from build123d import *

# Parameters (mm, degrees)
SKETCH_1_W               = 43.2
SKETCH_1_H               = 27.5
EXTRUDE_1_DEPTH          = 2
CUT_EXTRUDE_1_REACH      = 27.683
SKETCH_2_R               = 1.65
CUT_EXTRUDE_2_REACH      = 27.683
MIRROR_2_COPY_1_REACH    = 27.683
MIRROR_2_COPY_1_SKETCH_R = 1.65
MIRROR_2_COPY_2_REACH    = 27.683
CUT_EXTRUDE_3_REACH      = 27.683
SKETCH_4_R               = 4
SKETCH_5_W               = 5
SKETCH_5_H               = 24
EXTRUDE_2_DEPTH          = 19
CUT_EXTRUDE_5_REACH      = 50.159
SKETCH_6_R               = 6
CUT_EXTRUDE_6_REACH      = 35.115
SKETCH_7_R               = 1.65


with BuildPart() as part:
    # 草图1 → 凸台-拉伸1 (new body)
    with BuildSketch(Plane(origin=(0, 0, 0), x_dir=(1, 0, 0), z_dir=(0, 1, 0))):
        Rectangle(SKETCH_1_W, SKETCH_1_H)
    extrude(amount=EXTRUDE_1_DEPTH)

    # 草图2 → 切除-拉伸1 (cut, up to next)
    with BuildSketch(Plane(origin=(0, 2, 0), x_dir=(1, 0, 0), z_dir=(0, 1, 0)), mode=Mode.PRIVATE) as cut_extrude_1_sk1:
        with Locations(Location((-17, 9, 0), (0, 0, 270))):
            Circle(SKETCH_2_R)
    cut_extrude_1_tool1 = extrude(cut_extrude_1_sk1.sketch, amount=-CUT_EXTRUDE_1_REACH, mode=Mode.PRIVATE) & part.part
    cut_extrude_1 = cut_extrude_1_tool1.solids().sort_by_distance((-17, 2, -9))[0]
    add(cut_extrude_1, mode=Mode.SUBTRACT)

    # 草图3 → 切除-拉伸2 (cut, up to next)
    with BuildSketch(Plane(origin=(0, 2, 0), x_dir=(1, 0, 0), z_dir=(0, 1, 0)), mode=Mode.PRIVATE) as cut_extrude_2_sk1:
        with BuildLine():
            Line((-6.788225099, 4.5254834), (-10.033845225, 7.771103525))
            ThreePointArc((-10.033845225, 7.771103525), (-10.033845225, 10.033845225), (-7.771103525, 10.033845225))
            Line((-7.771103525, 10.033845225), (-4.5254834, 6.788225099))
            ThreePointArc((-4.5254834, 6.788225099), (-4.5254834, 4.5254834), (-6.788225099, 4.5254834))
        make_face()
    cut_extrude_2_tool1 = extrude(cut_extrude_2_sk1.sketch, amount=-CUT_EXTRUDE_2_REACH, mode=Mode.PRIVATE) & part.part
    cut_extrude_2 = cut_extrude_2_tool1.solids().sort_by_distance((-7.279664, 2, -7.279664))[0]
    add(cut_extrude_2, mode=Mode.SUBTRACT)

    # 镜向1: 切除-拉伸1, 切除-拉伸2 across plane
    add(cut_extrude_1.mirror(Plane.XY), mode=Mode.SUBTRACT)
    add(cut_extrude_2.mirror(Plane.XY), mode=Mode.SUBTRACT)

    # 镜向2: 切除-拉伸1, 切除-拉伸2 across plane
    add(cut_extrude_1.mirror(Plane(origin=(0, 0, 0), x_dir=(0, 0, 1), z_dir=(1, 0, 0))), mode=Mode.SUBTRACT)
    add(cut_extrude_2.mirror(Plane(origin=(0, 0, 0), x_dir=(0, 0, 1), z_dir=(1, 0, 0))), mode=Mode.SUBTRACT)

    # 镜向2 copy 1 sketch → 镜向2 copy 1 (cut, up to next)
    with BuildSketch(Plane(origin=(0, 2, 0), x_dir=(-1, 0, 0), z_dir=(0, 1, 0)), mode=Mode.PRIVATE) as mirror_2_copy_1_sk1:
        with Locations(Location((-17, 9, 0), (0, 0, 270))):
            Circle(MIRROR_2_COPY_1_SKETCH_R)
    mirror_2_copy_1_tool1 = extrude(mirror_2_copy_1_sk1.sketch, amount=-MIRROR_2_COPY_1_REACH, mode=Mode.PRIVATE) & part.part
    add(mirror_2_copy_1_tool1.solids().sort_by_distance((17, 2, 9))[0], mode=Mode.SUBTRACT)

    # 镜向2 copy 2 sketch → 镜向2 copy 2 (cut, up to next)
    with BuildSketch(Plane(origin=(0, 2, 0), x_dir=(-1, 0, 0), z_dir=(0, 1, 0)), mode=Mode.PRIVATE) as mirror_2_copy_2_sk1:
        with BuildLine():
            Line((-6.788225099, 4.5254834), (-10.033845225, 7.771103525))
            ThreePointArc((-10.033845225, 7.771103525), (-10.033845225, 10.033845225), (-7.771103525, 10.033845225))
            Line((-7.771103525, 10.033845225), (-4.5254834, 6.788225099))
            ThreePointArc((-4.5254834, 6.788225099), (-4.5254834, 4.5254834), (-6.788225099, 4.5254834))
        make_face()
    mirror_2_copy_2_tool1 = extrude(mirror_2_copy_2_sk1.sketch, amount=-MIRROR_2_COPY_2_REACH, mode=Mode.PRIVATE) & part.part
    add(mirror_2_copy_2_tool1.solids().sort_by_distance((7.279664, 2, 7.279664))[0], mode=Mode.SUBTRACT)

    # 草图4 → 切除-拉伸3 (cut, up to next)
    with BuildSketch(Plane(origin=(0, 2, 0), x_dir=(1, 0, 0), z_dir=(0, 1, 0)), mode=Mode.PRIVATE) as cut_extrude_3_sk1:
        with Locations(Location((0, 0, 0), (0, 0, 270))):
            Circle(SKETCH_4_R)
    cut_extrude_3_tool1 = extrude(cut_extrude_3_sk1.sketch, amount=-CUT_EXTRUDE_3_REACH, mode=Mode.PRIVATE) & part.part
    add(cut_extrude_3_tool1.solids().sort_by_distance((0, 2, 0))[0], mode=Mode.SUBTRACT)

    # 草图5 → 凸台-拉伸2 (add)
    with BuildSketch(Plane(origin=(0, 2, 0), x_dir=(1, 0, 0), z_dir=(0, 1, 0))):
        with Locations((-17, 0)):
            Rectangle(SKETCH_5_W, SKETCH_5_H)
    extrude_2 = extrude(amount=EXTRUDE_2_DEPTH)

    # 草图6 → 切除-拉伸5 (cut, up to next)
    with BuildSketch(Plane.ZY.offset(19.5), mode=Mode.PRIVATE) as cut_extrude_5_sk1:
        with Locations((0, 11.5)):
            Circle(SKETCH_6_R)
    cut_extrude_5_tool1 = extrude(cut_extrude_5_sk1.sketch, amount=-CUT_EXTRUDE_5_REACH, mode=Mode.PRIVATE) & part.part
    cut_extrude_5 = cut_extrude_5_tool1.solids().sort_by_distance((-19.5, 11.5, 0))[0]
    add(cut_extrude_5, mode=Mode.SUBTRACT)

    # 草图7 → 切除-拉伸6 (cut, up to next)
    with BuildSketch(Plane.XZ, mode=Mode.PRIVATE) as cut_extrude_6_sk1:
        with Locations(Location((-17, 9, 0), (0, 0, 270))):
            Circle(SKETCH_7_R)
    cut_extrude_6_tool1 = extrude(cut_extrude_6_sk1.sketch, amount=-CUT_EXTRUDE_6_REACH, mode=Mode.PRIVATE) & part.part
    # 草图7 → 切除-拉伸6 (cut, up to next)
    with BuildSketch(Plane.XZ, mode=Mode.PRIVATE) as cut_extrude_6_sk2:
        with Locations(Location((-17, -9, 0), (0, 0, 270))):
            Circle(SKETCH_7_R)
    cut_extrude_6_tool2 = extrude(cut_extrude_6_sk2.sketch, amount=-CUT_EXTRUDE_6_REACH, mode=Mode.PRIVATE) & part.part
    add(cut_extrude_6_tool1.solids().sort_by_distance((-17, 0, 9))[0], mode=Mode.SUBTRACT)
    add(cut_extrude_6_tool2.solids().sort_by_distance((-17, 0, -9))[0], mode=Mode.SUBTRACT)

    # 镜向3: 切除-拉伸1, 凸台-拉伸2, 切除-拉伸5 across plane
    add(cut_extrude_1.mirror(Plane(origin=(0, 0, 0), x_dir=(0, 0, 1), z_dir=(1, 0, 0))), mode=Mode.SUBTRACT)
    add(extrude_2.mirror(Plane(origin=(0, 0, 0), x_dir=(0, 0, 1), z_dir=(1, 0, 0))))
    add(cut_extrude_5.mirror(Plane(origin=(0, 0, 0), x_dir=(0, 0, 1), z_dir=(1, 0, 0))), mode=Mode.SUBTRACT)


solid = part.part
CAD build for the part. Positions are in the model's coordinates, mm. A direction names the side the tool comes from. Coordinates: 2 decimals unless noted, no trailing zeros. Write each loop counter-clockwise with the first axis right and the second up, starting at its lowest first coordinate (ties: lowest second). Pieces come first, ordered by that corner, then holes. Notation, with made-up numbers: M 8,75 L 13,75 A19 ccw 13,81 Z; hole C 48.5,77.25 d8. An arc over 180 degrees is marked long. Answer as a JSON object with one key per item and string values. Group by question number.
1) Saw through at A-A (x = 0). Write the cut outline in (y, z), plus the area to 3 significant figures.
2) Tool access for faces 1 (the face through (14.5, 5, 0)), 2 (the face through (17, 2, -9)), 3 (the face through (-17, 11, 12)), 4 (the face through (-8.39, 1.01, 6.13)): list every direction of +Z, -Z, +X, -X, +Y, -Y with a clear straight run to the whole face (end or side of a thin tool).
3) Saw through at D-D (z = 0). Write the cut outline in (x, y), plus the area to 3 significant figures.
4) Mould opens along Z. For faces 5 (the face through (17, 11, 12)), 6 (the face through (-17, 11, -12)), 7 (the face through (15.885, 1.014, 10.216)), 8 (the face through (-19.5, 5, 0)) say: +Z half, -Z half, draft (parallel to the pull), parting line (faces both ways), or undercut.
5) Saw through at B-B (y = 11.5). Write the cut outline in (x, z), plus the area to 3 significant figures.
6) Saw through at C-C (x = -17). Write the cut outline in (y, z), plus the area to 3 significant figures.
7) Wall check: line 1 (Z direction, x = 17, y = 0.75); line 2 (X direction, y = 11.75, z = 9); line 3 (X direction, y = 7, z = 4.5). Give the ranges that are in metal, low to high. Write a range as from..to.
8) Pin check, flat tips, straight feed: pin 1 Ø3 at (y, z) = (4, -9) entering from -X; pin 2 Ø1 at (x, z) = (17.5, -9) entering from -Y; pin 3 Ø5.5 at (y, z) = (15.5, 4) entering from +X; pin 4 Ø1.5 at (x, y) = (-13.5, 12) entering from -Z. Stop position of each tip, or through.
Values follow:
{
 "1": {"outline": "M 0,-13.75 L 2,-13.75 L 2,-4 L 0,-4 Z; M 0,4 L 2,4 L 2,13.75 L 0,13.75 Z", "area": "39.0 mm2"},
 "2": {"face 1": "+Z, -Z, +Y", "face 2": "-Y", "face 3": "+Z, +X, -X, +Y", "face 4": "+Y, -Y"},
 "3": {"outline": "M -21.6,0 L -4,0 L -4,2 L -14.5,2 L -14.5,5.5 L -19.5,5.5 L -19.5,2 L -21.6,2 Z; M -19.5,17.5 L -14.5,17.5 L -14.5,21 L -19.5,21 Z; M 4,0 L 21.6,0 L 21.6,2 L 19.5,2 L 19.5,5.5 L 14.5,5.5 L 14.5,2 L 4,2 Z; M 14.5,17.5 L 19.5,17.5 L 19.5,21 L 14.5,21 Z", "area": "140 mm2"},
 "4": {"face 5": "+Z half", "face 6": "-Z half", "face 7": "undercut", "face 8": "draft"},
 "5": {"outline": "M -19.5,-12 L -14.5,-12 L -14.5,-6 L -19.5,-6 Z; M -19.5,6 L -14.5,6 L -14.5,12 L -19.5,12 Z; M 14.5,-12 L 19.5,-12 L 19.5,-6 L 14.5,-6 Z; M 14.5,6 L 19.5,6 L 19.5,12 L 14.5,12 Z; hole C -17,-9 d3.3; hole C -17,9 d3.3", "area": "103 mm2"},
 "6": {"outline": "M 0,-13.75 L 2,-13.75 L 2,-12 L 21,-12 L 21,-10.65 L 0,-10.65 Z; M 0,-7.35 L 21,-7.35 L 21,7.35 L 0,7.35 Z; M 0,10.65 L 21,10.65 L 21,12 L 2,12 L 2,13.75 L 0,13.75 Z; hole C 11.5,0 d12", "area": "259 mm2"},
 "7": {"line 1": "z = -13.75..-10.65, -7.35..7.35, 10.65..13.75", "line 2": "x = -19.5..-18.65, -15.35..-14.5, 14.5..19.5", "line 3": "x = -19.5..-14.5, 14.5..19.5"},
 "8": {"pin 1": "stops at x = -19.5", "pin 2": "stops at y = 2", "pin 3": "stops at x = 19.5", "pin 4": "passes through"}
}
